from build123d import *

# Parameters (mm, degrees)
BOSS_EXTRUDE1_DEPTH             = 40
SKETCH2_W                       = 65
SKETCH2_H                       = 10
CUT_EXTRUDE1_DEPTH              = 35
CUT_EXTRUDE2_DEPTH              = 40
SKETCH4_W                       = 55
SKETCH4_H                       = 10
CUT_EXTRUDE3_DEPTH              = 98.114622998
CHAMFER1_SIZE                   = 5
SKETCH5_W                       = 40
SKETCH5_H                       = 120
BOSS_EXTRUDE2_DEPTH             = 15
SKETCH16_W                      = 40
SKETCH16_H                      = 40
BOSS_EXTRUDE4_DEPTH             = 10
SKETCH6_R                       = 4.15
CUT_EXTRUDE4_DEPTH              = 115
CHAMFER2_SIZE                   = 1
FILLET1_R                       = 10
FILLET2_R                       = 5
SKETCH9_W                       = 40
SKETCH9_H                       = 40
BOSS_EXTRUDE3_DEPTH             = 40
FILLET3_R                       = 10
SKETCH10_R                      = 8
CUT_EXTRUDE6_DEPTH              = 20
SKETCH11_R                      = 4.5
CUT_EXTRUDE7_DEPTH              = 30
SKETCH12_R                      = 4.15
CUT_EXTRUDE8_DEPTH              = 100
CHAMFER7_SIZE                   = 1
FILLET5_R                       = 10
CHAMFER10_SIZE                  = 3
CHAMFER11_SIZE                  = 2
FILLET6_R                       = 10
CHAMFER13_SIZE                  = 3
F_1_5MM_DOWEL_HOLE1_D           = 1.5
F_1_5MM_DOWEL_HOLE1_DEPTH       = 20
F_1_5MM_DOWEL_HOLE1_CSINK_D     = 1.55
F_1_5MM_DOWEL_HOLE1_CSINK_ANGLE = 90
F_1_5MM_DOWEL_HOLE1_TIP         = 0.450645464


# Some blends are built 0.0001 mm under size
with BuildPart() as part:
    # Sketch1 → Boss-Extrude1 (new body)
    with BuildSketch(Plane(origin=(0, 0, 0), x_dir=(0, 0, -1), z_dir=(1, 0, 0))):
        Polygon((37.5, 30), (37.5, 50), (-57.5, 50), (-57.5, -70), (37.5, -70), (37.5, -30), (-37.5, -30), (-37.5, 30), align=None)
    extrude(amount=BOSS_EXTRUDE1_DEPTH)

    # Sketch2 → Cut-Extrude1 (cut)
    with BuildSketch(Plane(origin=(40, 0, 0), x_dir=(0, 0, -1), z_dir=(1, 0, 0))):
        with Locations((0, -45)):
            Rectangle(SKETCH2_W, SKETCH2_H)
    extrude(amount=-CUT_EXTRUDE1_DEPTH, mode=Mode.SUBTRACT)

    # Sketch3 → Cut-Extrude2 (cut)
    with BuildSketch(Plane.XZ.offset(70)):
        with BuildLine():
            Line((9.5, -11.401754251), (9.5, 11.401754251))
            ThreePointArc((9.5, 11.401754251), (20, 15.5), (30.5, 11.401754251))
            Line((30.5, 11.401754251), (30.5, -11.401754251))
            ThreePointArc((30.5, -11.401754251), (20, -15.5), (9.5, -11.401754251))
        make_face()
    extrude(amount=-CUT_EXTRUDE2_DEPTH, mode=Mode.SUBTRACT)

    # Sketch4 → Cut-Extrude3 (cut, through all)
    with BuildSketch(Plane(origin=(5, 0, 0), x_dir=(0, 0, -1), z_dir=(1, 0, 0))):
        with Locations((0, -45)):
            Rectangle(SKETCH4_W, SKETCH4_H)
    extrude(amount=-CUT_EXTRUDE3_DEPTH, mode=Mode.SUBTRACT)

    # Chamfer1
    chamfer1_edges = [part.edges().sort_by_distance(p)[0] for p in [
        (5, -45, 27.5),
        (5, -45, -27.5),
    ]]
    chamfer(chamfer1_edges, length=CHAMFER1_SIZE - 0.0001)  # a hair under: the kernel refuses the full size

    # Sketch5 → Boss-Extrude2 (add)
    with BuildSketch(Plane.XY.offset(57.5)):
        with Locations((20, -10)):
            Rectangle(SKETCH5_W, SKETCH5_H)
    extrude(amount=BOSS_EXTRUDE2_DEPTH)

    # Sketch16 → Boss-Extrude4 (add)
    with BuildSketch(Plane(origin=(0, 0, -37.5), x_dir=(-1, 0, 0), z_dir=(0, 0, -1))):
        with Locations((-20, -50)):
            Rectangle(SKETCH16_W, SKETCH16_H)
    extrude(amount=BOSS_EXTRUDE4_DEPTH)

    # Sketch6 → Cut-Extrude4 (cut)
    with BuildSketch(Plane.XZ.offset(70)):
        with Locations(Location((30, 57.5, 0), (0, 0, 270))):
            Circle(SKETCH6_R)
        with Locations(Location((10, 57.5, 0), (0, 0, 270))):
            Circle(SKETCH6_R)
    extrude(amount=-CUT_EXTRUDE4_DEPTH, mode=Mode.SUBTRACT)

    # Chamfer2
    chamfer2_edges = [part.edges().sort_by_distance(p)[0] for p in [
        (30, -70, 61.65),
        (10, -70, 61.65),
    ]]
    chamfer(chamfer2_edges, length=CHAMFER2_SIZE)

    # Fillet1
    # the kernel refuses this fillet: 10 mm, written as the material it takes off along each edge
    with BuildSketch(Plane(origin=(-25, -70, -47.5), x_dir=(0, 0, 1), z_dir=(1, 0, 0))) as fillet1_piece_1:
        with BuildLine():
            CenterArc((FILLET1_R, -FILLET1_R), FILLET1_R, 90, 90)
            Line((0, -FILLET1_R), (0, 0))
            Line((0, 0), (FILLET1_R, 0))
        make_face()
    extrude(amount=90, mode=Mode.SUBTRACT)
    with BuildSketch(Plane(origin=(65, -30, -47.5), x_dir=(0, -1, 0), z_dir=(-1, 0, 0)), Plane(origin=(-25, -70, 72.5), x_dir=(0, 0, -1), z_dir=(1, 0, 0))) as fillet1_piece_2:
        with BuildLine():
            CenterArc((FILLET1_R, FILLET1_R), FILLET1_R, 180, 90)
            Line((0, FILLET1_R), (0, 0))
            Line((0, 0), (FILLET1_R, 0))
        make_face()
    extrude(amount=90, mode=Mode.SUBTRACT)

    # Fillet2
    fillet2_edges = [part.edges().sort_by_distance(p)[0] for p in [
        (20, 30, 37.5),
        (20, -30, 37.5),
    ]]
    fillet(fillet2_edges, radius=FILLET2_R)

    # Sketch9 → Boss-Extrude3 (add)
    with BuildSketch(Plane(origin=(0, 50, 0), x_dir=(1, 0, 0), z_dir=(0, 1, 0))):
        with Locations((20, -52.5)):
            Rectangle(SKETCH9_W, SKETCH9_H)
    extrude(amount=BOSS_EXTRUDE3_DEPTH)

    # Fillet3
    fillet3_edges = [part.edges().sort_by_distance(p)[0] for p in [
        (0, 90, 52.5),
        (40, 90, 52.5),
    ]]
    fillet(fillet3_edges, radius=FILLET3_R)

    # Sketch10 → Cut-Extrude6 (cut)
    with BuildSketch(Plane(origin=(0, 0, 72.5), x_dir=(-1, 0, 0), z_dir=(0, 0, -1))):
        with Locations((-20, 70)):
            Circle(SKETCH10_R)
    extrude(amount=CUT_EXTRUDE6_DEPTH, mode=Mode.SUBTRACT)

    # Sketch11 → Cut-Extrude7 (cut)
    with BuildSketch(Plane.XY.offset(52.5)):
        with Locations((20, 70)):
            Circle(SKETCH11_R)
    extrude(amount=-CUT_EXTRUDE7_DEPTH, mode=Mode.SUBTRACT)

    # Sketch12 → Cut-Extrude8 (cut)
    with BuildSketch(Plane.XY.offset(72.5)):
        with Locations((20, 40)):
            Circle(SKETCH12_R)
    extrude(amount=-CUT_EXTRUDE8_DEPTH, mode=Mode.SUBTRACT)

    # Chamfer7
    chamfer7_edges = [part.edges().sort_by_distance(p)[0] for p in [
        (15.85, 40, 72.5),
    ]]
    chamfer(chamfer7_edges, length=CHAMFER7_SIZE)

    # Fillet5
    fillet5_edges = [part.edges().sort_by_distance(p)[0] for p in [
        (20, 30, -37.5),
    ]]
    fillet(fillet5_edges, radius=FILLET5_R)

    # Chamfer10
    chamfer10_edges = [part.edges().sort_by_distance(p)[0] for p in [
        (28, 70, 72.5),
    ]]
    chamfer(chamfer10_edges, length=CHAMFER10_SIZE)

    # Chamfer11
    chamfer11_edges = [part.edges().sort_by_distance(p)[0] for p in [
        (15.5, 70, 32.5),
    ]]
    chamfer(chamfer11_edges, length=CHAMFER11_SIZE)

    # Fillet6
    fillet6_edges = [part.edges().sort_by_distance(p)[0] for p in [
        (20, 50, -37.5),
    ]]
    fillet(fillet6_edges, radius=FILLET6_R - 0.0001)  # a hair under: the kernel refuses the full size

    # Chamfer13
    chamfer13_edges = [part.edges().sort_by_distance(p)[0] for p in [
        (40, -50, -47.5),
        (0, -50, -47.5),
        (0, -30, -2.5),
        (0, -70, 12.5),
        (0, -67.071067812, 69.571067812),
        (0, -32.928932188, -44.571067812),
        (0, -67.071067812, -44.571067812),
        (40, -70, 12.5),
        (40, 10, 72.5),
        (40, -30, -2.5),
        (40, -67.071067812, 69.571067812),
        (40, -32.928932188, -44.571067812),
        (40, -67.071067812, -44.571067812),
        (0, 0, 37.5),
        (40, 0, 37.5),
        (0, 30, 2.5),
        (40, 30, 2.5),
        (0, -28.535533906, 36.035533906),
        (40, -28.535533906, 36.035533906),
        (0, 28.535533906, 36.035533906),
        (40, 28.535533906, 36.035533906),
        (20, 90, 72.5),
        (20, 90, 32.5),
        (0, 10, 72.5),
        (37.071067812, 87.071067812, 72.5),
        (2.928932188, 87.071067812, 72.5),
        (0, 65, 32.5),
        (40, 65, 32.5),
        (37.071067812, 87.071067812, 32.5),
        (2.928932188, 87.071067812, 32.5),
        (0, 32.928932188, -34.571067812),
        (40, 32.928932188, -34.571067812),
        (40, 50, 2.49995),
        (0, 50, 2.49995),
        (0, 47.071097101, -34.571097101),
        (40, 47.071097101, -34.571097101),
    ]]
    chamfer(chamfer13_edges, length=CHAMFER13_SIZE)

    # Ø1.5mm Dowel Hole1
    with Locations(Plane(origin=(0, 0, 32.5), x_dir=(-1, 0, 0), z_dir=(0, 0, -1))):
        with Locations((-29.526279442, 64.5), (-20, 81), (-10.473720558, 64.5), (-20, 70)):
            CounterSinkHole(F_1_5MM_DOWEL_HOLE1_D / 2, F_1_5MM_DOWEL_HOLE1_CSINK_D / 2, depth=F_1_5MM_DOWEL_HOLE1_DEPTH, counter_sink_angle=F_1_5MM_DOWEL_HOLE1_CSINK_ANGLE)
            with Locations((0, 0, -(F_1_5MM_DOWEL_HOLE1_DEPTH + F_1_5MM_DOWEL_HOLE1_TIP / 2))):  # 118° drill point
                Cone(0, F_1_5MM_DOWEL_HOLE1_D / 2, F_1_5MM_DOWEL_HOLE1_TIP, mode=Mode.SUBTRACT)


solid = part.part
Model file for the job. Use its own axes, mm. A direction names the side the tool comes from. Coordinates: 2 decimals unless noted, no trailing zeros. Order: outer loops, then holes, each group sorted by start corner. A loop starts at its lowest first (then second) coordinate and runs counter-clockwise, first axis right, second up. Notation, with made-up numbers: (-38.5, -4) -> (-1.5, -4) arc R11 cw to (-1.5, 6) -> close; hole circle Ø7 at (6, 29.25). An arc over 180 degrees is marked (long way). Return JSON: item names as keys, results as strings. Group by question number.
Item 1: Flat gauge pins, fed straight in: P1, Ø1, axis at x = 24, z = -14, coming from the +Y side; P2, Ø14.5, axis at x = 20, y = 70, coming from the -Z side; P3, Ø17.5, axis at x = 21.5, y = 68.5, coming from the +Z side. Where does each tip first touch, or does it go through?
Item 2: Saw through at C-C on y = -10. Write the cut outline in (x, z).
Item 3: Wall check: line 1 along Y through (x, z) = (20, 38); line 2 along X through (y, z) = (64.5, 37); line 3 along Y through (x, z) = (20, 53). Give the ranges that are in metal, low to high. Write a range as [from, to].
Item 4: Tool access for faces 4 (the cylindrical face through (19.46, 44.115, 22.693)), 5 (the conical face through (1.146, 34.304, -33.323)), 6 (the cylindrical face through (19.8, -35.1, 15.5)), 7 (the flat face through (34, -50, 0)), 8 (the flat face through (20, 50, 2)): list every direction of +Z, -Z, +X, -X, +Y, -Y with a clear straight run to the whole face (end or side of a thin tool).
Item 5: Saw through at D-D on y = 55.5. Write the cut outline in (x, z), then the cut area to 3 significant figures.
Item 6: Saw through at A-A on y = -47. State how many separate pieces and enclosed holes the cut face has, then the cut area to 3 significant figures.
Item 7: Pull direction X, two halves, no side cores. Call faces 1 (the flat face through (10, 45, 58)), 2 (the flat face through (20, 30, 3)), 3 (the flat face through (2.5, -45.1, -30)): pulls with the +X half, pulls with the -X half, needs draft (parallel to the pull), parting line crosses it, or undercut.
Values found:
{
 "1": {"P1": "stops at y = 50", "P2": "stops at z = 32.5", "P3": "stops at z = 72.37"},
 "2": {"outline": "(0, 40.5) -> (3, 37.5) -> (37, 37.5) -> (40, 40.5) -> (40, 69.5) -> (37, 72.5) -> (3, 72.5) -> (0, 69.5) -> close; hole circle Ø8.3 at (10, 57.5); hole circle Ø8.3 at (30, 57.5)"},
 "3": {"line 1": "y = [-70, 35.85], [44.15, 65.5], [74.5, 80.25], [81.75, 90]", "line 2": "x = [0, 9.72], [11.22, 28.78], [30.28, 40]", "line 3": "y = [-70, 35.85], [44.15, 62], [78, 90]"},
 "4": {"face 4": "+Z", "face 5": "-Z, -X", "face 6": "-Y", "face 7": "+X", "face 8": "-Z, +X, -X, +Y"},
 "5": {"outline": "(0, 35.5) -> (3, 32.5) -> (37, 32.5) -> (40, 35.5) -> (40, 69.5) -> (37, 72.5) -> (3, 72.5) -> (0, 69.5) -> close", "area": "1,580 mm2"},
 "6": {"separate pieces": "2", "enclosed holes": "2", "area": "2,100 mm2"},
 "7": {"face 1": "undercut", "face 2": "needs draft", "face 3": "pulls with the +X half"}
}
